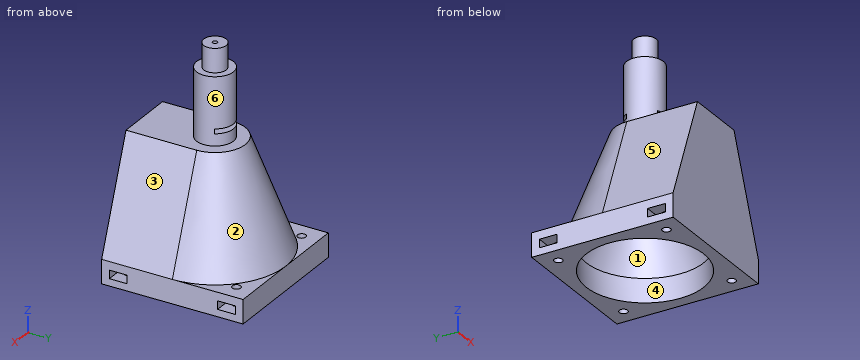
Autodesk Inventor part; units mm, degrees
ref_plane "YZ Plane" through (0, 0, 0) normal (1, 0, 0) x (0, 1, 0)
ref_plane "XZ Plane" through (0, 0, 0) normal (0, 1, 0) x (-1, 0, 0)
sketch "Sketch2" plane through (0, 0, 0) normal (0, 0, 1) x (1, 0, 0)
  line L0 (-29.75, 59.5) -> (29.75, 59.5)
  line L1 (29.75, 59.5) -> (29.75, 0)
  line L2 (29.75, 0) -> (-29.75, 0)
  line L3 (-29.75, 0) -> (-29.75, 59.5)
  point P0 (0, 0)
  point P1 (0, 0)
  dimension "d0" = 59.5
extrude "Extrusion1" add sketch "Sketch2" along normal blind 55
sketch "Sketch3" plane through (0, 0, 55) normal (0, 0, 1) x (1, 0, 0)
  circle A0 centre (0, 29.75) radius 1
  circle A1 centre (0, 29.75) radius 7.75
  line L0 (0, 0) -> (0, 59.5) construction
  line L1 (29.75, 59.5) -> (-29.75, 59.5) construction
  line L2 (29.75, 0) -> (29.75, 59.5) construction
  line L3 (29.75, 29.75) -> (-29.75, 29.75) construction
  line L4 (-29.75, 59.5) -> (-29.75, 0) construction
  line L5 (-29.75, 0) -> (29.75, 0)
  dimension "d3" = 15.5
  dimension "d5" = 2
  dimension "d47" = 22
extrude "Extrusion2" add sketch "Sketch3" along normal blind 28.3
sketch "Sketch4" plane through (0, 29.75, 83.3) normal (0, 0, 1) x (1, 0, 0)
  circle A0 centre (0, 0) radius 1
  circle A1 centre (0, 0) radius 4.75
  circle A2 centre (0, 0) radius 1
  point P0 (0, -29.75)
  dimension "d8" = 9.5
extrude "Extrusion3" add sketch "Sketch4" along normal blind 10
sketch "Sketch10" plane through (0, 0, 0) normal (0, 0, -1) x (-1, 0, 0)
  circle A0 centre (-22.75, 52.5) radius 1.75
  circle A1 centre (-22.75, 7) radius 1.75
  circle A2 centre (22.75, 52.5) radius 1.75
  circle A3 centre (22.75, 7) radius 1.75
  line L0 (-29.75, 59.5) -> (-29.75, 0)
  line L1 (29.75, 59.5) -> (-29.75, 59.5)
  line L2 (-29.75, 29.75) -> (29.75, 29.75) construction
  line L3 (29.75, 0) -> (29.75, 59.5) construction
  line L4 (0, 59.5) -> (0, 0) construction
  dimension "d29" = 7
  dimension "d30" = 7
  dimension "d33" = 3.5
extrude "Extrusion5" cut sketch "Sketch10" against normal blind 10
sketch "Sketch9" plane through (29.75, 0, 0) normal (1, 0, 0) x (0, 0, -1)
  line L0 (-6.5, 56.25) -> (-3, 56.25)
  line L1 (-3, 56.25) -> (-3, 48.75)
  line L2 (-3, 48.75) -> (-6.5, 48.75)
  line L3 (-6.5, 48.75) -> (-6.5, 56.25)
  line L4 (-6.5, 10.75) -> (-3, 10.75)
  line L5 (-3, 10.75) -> (-3, 3.25)
  line L6 (-3, 3.25) -> (-6.5, 3.25)
  line L7 (-6.5, 3.25) -> (-6.5, 10.75)
  line L8 (0, 59.5) -> (-55, 59.5)
  line L9 (-55, 0) -> (-55, 59.5) construction
  line L10 (-55, 29.75) -> (0, 29.75) construction
  line L11 (0, 0) -> (0, 59.5) construction
  line L12 (0, 54.25) -> (0, 50.75)
  line L13 (0, 52.5) -> (-10, 52.5) construction
  line L14 (-10, 54.25) -> (-10, 50.75)
  dimension "d24" = 7.5
  dimension "d25" = 3.5
  dimension "d26" = 3
extrude "Extrusion4" cut sketch "Sketch9" against normal blind 10
mirror "Mirror1" about plane through (0, 0, 0) normal (1, 0, 0) of "Extrusion4"
ref_plane "Work Plane1" through (0, 0, 10) normal (0, 0, 1) x (1, 0, 0)
sketch "Sketch11" plane through (0, 0, 10) normal (0, 0, 1) x (1, 0, 0)
  circle A0 centre (0, 29.75) radius 24.75
  circle A1 centre (0, 29.75) radius 1
  line L0 (-29.75, 59.5) -> (29.75, 59.5)
  point P0 (0, 0)
  dimension "d49" = 5
extrude "Extrusion6" cut sketch "Sketch11" against normal through all contours A0 | A1
loft "Loft2" cut section 1 edges at (-24.75, 29.75, 10) section 2 edges at (-1, 29.75, 55)
sketch "Sketch7" plane through (-29.75, 59.5, 0) normal (0, 1, 0) x (1, 0, 0)
  line L0 (36.5, -60) -> (23, -60)
  line L1 (23, -60) -> (23, -62)
  line L2 (23, -62) -> (36.5, -62)
  line L3 (36.5, -62) -> (36.5, -60)
  line L4 (29.75, -60) -> (29.75, -62) construction
  line L5 (26.5, -55) -> (28.5, -55) construction
  line L6 (29.75, -55) -> (29.75, -83.3) construction
  line L7 (59.5, -55) -> (0, -55) construction
  line L8 (22, -83.3) -> (37.5, -83.3)
  point P0 (29.75, 0)
  dimension "d16" = 2
  dimension "d17" = 13.5
  dimension "d18" = 5
extrude "Extrusion7" cut sketch "Sketch7" against normal blind 32
sketch "Sketch12" plane through (-29.75, 27.5, 0) normal (0, 1, 0) x (1, 0, 0)
  line L0 (32.75, -60) -> (26.75, -60)
  line L1 (26.75, -60) -> (26.75, -62)
  line L2 (26.75, -62) -> (32.75, -62)
  line L3 (32.75, -62) -> (32.75, -60)
  line L4 (36.5, -60) -> (36.5, -62)
  line L5 (36.5, -62) -> (23, -62)
  line L6 (28.75, -60) -> (30.75, -60) construction
  line L7 (29.75, -60) -> (29.75, -62) construction
  line L8 (30.75, -62) -> (28.75, -62) construction
  point P0 (29.75, 0)
  point P1 (22.3338, -63)
  dimension "d44" = 6
extrude "Extrusion8" cut sketch "Sketch12" against normal through all
sketch "Sketch14" plane through (0, 0, 0) normal (1, 0, 0) x (0, 1, 0)
  line L0 (59.5, 10) -> (42.5, 55)
  line L1 (42.5, 55) -> (79.5, 55)
  line L2 (79.5, 10) -> (79.5, 55)
  line L3 (59.5, 55) -> (0, 55)
  line L4 (37.5, 55) -> (37.5, 83.3)
  line L5 (59.5, 0) -> (59.5, 55)
  line L6 (5, 10) -> (54.5, 10)
  line L7 (79.5, 10) -> (59.5, 10)
  line L8 (59.5, 0) -> (59.5, 55)
  line L9 (54.25, 10) -> (50.75, 10)
  line L10 (29.75, -18.66) -> (29.75, 111.96)
  point P0 (0, 0)
  point P1 (55, 37.5)
  point P2 (55, 37.5)
  dimension "d54" = 5
  dimension "d55" = 20
revolve "Revolution1" cut sketch "Sketch14" angle 180 mid plane about axis through (0, 29.75, 55) along (0, 0, 1)
sketch "Sketch15" plane through (12.75, 29.75, 55) normal (0, 1, 0) x (1, 0, 0)
  line L0 (-42.5, 0) -> (-25.5, 0)
  line L1 (-25.5, 0) -> (0, 0)
  line L2 (-42.5, 0) -> (17, 0)
  line L3 (0, 0) -> (17, 0)
  line L4 (17, 0) -> (17, 45)
  line L5 (17, 55) -> (17, 0)
  line L6 (0, 0) -> (17, 45)
  line L7 (0, 0) -> (17, 45)
  line L8 (17, 45) -> (-25.5, 0)
  line L9 (-25.5, 0) -> (-42.5, 45)
  line L10 (-42.5, 45) -> (-25.5, 0)
  line L11 (-42.5, 0) -> (-42.5, 45)
  line L12 (-42.5, 55) -> (-42.5, 0)
  point P0 (-12.75, 55)
extrude "Extrusion10" cut sketch "Sketch15" against normal through all contours L11 L9 L0 | L6 L4 L2
properties part number "Power_Meter_Adapter_Part1"
Build history of the part. All positions in model axes, mm. Face numbers are marked on the shaded views. A direction names the side the tool comes from. Give positions to 0.01 mm unless a question says otherwise; leave off trailing zeros. Loops run counter-clockwise (first coordinate to the right, second up) from the corner with the lowest first, then second, coordinate; pieces in that order, holes last. Notation, with made-up numbers: (0.25, 51.5) -> (36.25, 51.5) arc R20 ccw to (36.25, 62.5) -> close; hole circle Ø5 at (89.5, 48.5). An arc over 180 degrees is marked (long way). Answer in a Markdown table with one row per item.
Item 1: Slice it at D-D on z = 70.5. Write the cut outline in (x, y), plus the area to 3 significant figures.
Findings below:
| item | result |
|---|---|
| outline | circle Ø15.5 at (0, 29.75); hole circle Ø2 at (0, 29.75) |
| area | 186 mm² |
Item 2: Tool access for the marked faces 5 and 6: list every direction of +Z, -Z, +X, -X, +Y, -Y with a clear straight run to the whole face (end or side of a thin tool).
Findings below:
| item | result |
|---|---|
| face 5 | +Z, -X, +Y, -Y |
| face 6 | +Z |
Item 3: Slice it at A-A on z = 51.5. Write the cut outline in (x, y).
Findings below:
| item | result |
|---|---|
| outline | (-14.07, 0) -> (14.07, 0) -> (14.07, 29.75) arc R14.07 ccw to (-14.07, 29.75) -> close; hole circle Ø5.69 at (0, 29.75) |
Item 4: Slice it at B-B on y = 7. Give the number of separate pieces and of enclosed holes in the cut face, plus the area to 3 significant figures.
Findings below:
| item | result |
|---|---|
| separate pieces | 3 |
| enclosed holes | 0 |
| area | 2,150 mm² |
Item 5: Mould opens along Y. For the marked faces 1, 2, 3 and 4 say: pulls with the +Y half, pulls with the -Y half, needs draft (parallel to the pull), parting line crosses it, or undercut.
Findings below:
| item | result |
|---|---|
| face 1 | undercut |
| face 2 | pulls with the +Y half |
| face 3 | needs draft |
| face 4 | undercut |
Item 6: Flat gauge pins, fed straight in: P1, Ø6, axis at x = -13.5, z = 22, coming from the +Y side; P2, Ø1, axis at y = 22, z = 19.5, coming from the +X side; P3, Ø12, axis at x = -4.5, z = 82.5, coming from the +Y side. Where does each tip first touch, or does it go through?
Findings below:
| item | result |
|---|---|
| P1 | stops at y = 53.15 |
| P2 | stops at x = 26.35 |
| P3 | stops at y = 37.5 |
Item 7: Probe line 1 along Y through (x, z) = (0, 83); line 2 along Y through (x, z) = (-22.75, 8); line 3 along Y through (x, z) = (22, 7). List the from-to ranges inside material, lowest first. Write a range as [from, to].
Findings below:
| item | result |
|---|---|
| line 1 | y = [22, 28.75], [30.75, 37.5] |
| line 2 | y = [0, 5.25], [8.75, 20], [39.5, 50.75], [54.25, 59.5] |
| line 3 | y = [0, 5.42], [8.58, 18.41], [41.09, 50.92], [54.08, 59.5] |
